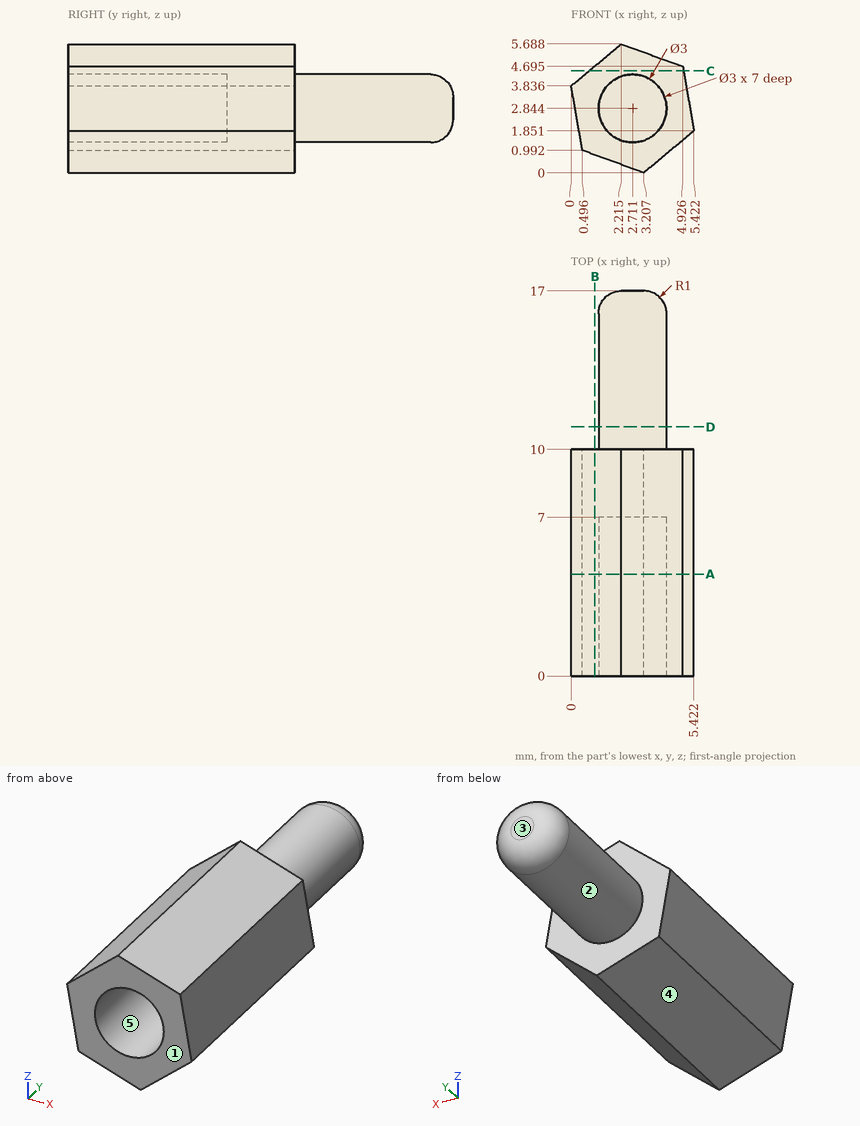
Here's the drawing with two shaded views (mm, measured from the low corner). I have some questions. A direction names the side the tool comes from. Give positions to 0.01 mm unless a question says otherwise; leave off trailing zeros. Write each loop counter-clockwise with the first axis right and the second up, starting at its lowest first coordinate (ties: lowest second). Pieces come first, ordered by that corner, then holes. Notation, with made-up numbers: (-20.5, 9.25) - (-11.5, 9.25) arc R9 cw to (-11.5, 17.25) - close; hole circle Ø11 at (20.25, 60.5). An arc over 180 degrees is marked (long way). Write item = value, one per line. Start each with the question number.
1. Imagine slicing it at D-D (y = 11). Please give me the cut outline in (x, z).
2. Please list where these lines run through material, in increasing order: line 1 (Y direction, x = 4.2, z = 1.9); line 2 (X direction, y = 6.5, z = 2.1) (1 decimal); line 3 (X direction, y = 6.25, z = 1.5) (1 decimal).
3. Imagine slicing it at B-B (x = 1.05). Please give me the cut outline in (y, z).
4. For pin 1 (3 mm diameter, centred on x = 5, z = 1.5, fed in from -Y); pin 2 (1.5 mm diameter, centred on y = 7, z = 2.5, fed in from -X), each with a flat end and sliding along its axis, tell me the tip position at first contact or that it passes through.
5. Imagine slicing it at C-C (z = 4.5). Please give me the cut outline in (x, y) (1 decimal).
6. On a 3-axis mill with a long thin cutter (end or side, diameter ignored), from which of +Z, -Z, +X, -X, +Y, -Y can I reach the whole of each face in a straight line? I mean the marked faces 1 and 2. Say none if no direction works.
7. Thinking about a two-plate mould opening in Z: for the marked faces 3, 4 and 5, which applies, released by +Z, released by -Z, zero draft, split by the parting line, or undercut?
8. Imagine slicing it at A-A (y = 4.5). Please give me the cut outline in (x, z) (1 decimal), and give its area (3 significant figures).
Worked answers:
q1.outline = circle Ø3 at (2.71, 2.84)
q2.line_1 = 0 to 10
q2.line_2 = 0.3 to 1.4, 4 to 5.4
q2.line_3 = 0.4 to 2, 3.4 to 5
q3.outline = (0, 0.79) - (10, 0.79) - (10, 4.71) - (0, 4.71) - close
q4.pin_1 = 0
q4.pin_2 = 0.1
q5.outline = (0.8, 0) - (5, 0) - (5, 10) - (0.8, 10) - close
q6.face_1 = +Z, -Z, +X, -X, -Y
q6.face_2 = +Y
q7.face_3 = zero draft
q7.face_4 = released by -Z
q7.face_5 = undercut
q8.outline = (0, 3.8) - (0.5, 1) - (3.2, 0) - (5.4, 1.9) - (4.9, 4.7) - (2.2, 5.7) - close; hole circle Ø3 at (2.7, 2.8)
q8.area = 14.6 mm2
